Answer from the drawing. Dimensions are ordinates in mm from the lowest x, y and z of the part. A direction names the side the tool comes from. Coordinates: 2 decimals unless noted, no trailing zeros. Write each loop counter-clockwise with the first axis right and the second up, starting at its lowest first coordinate (ties: lowest second). Pieces come first, ordered by that corner, then holes. Notation, with made-up numbers: (26.25, 67.5) -> (40.25, 67.5) arc R18 ccw to (40.25, 78.5) -> close; hole circle Ø4 at (58, 36). An arc over 180 degrees is marked (long way). Return JSON: item names as keys, results as strings.
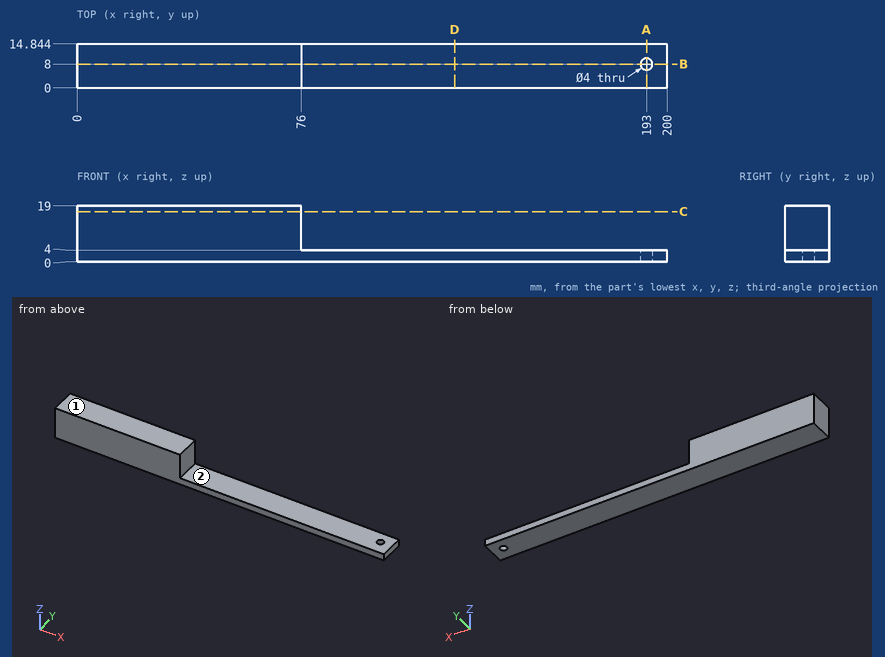
1. Consider L1, parallel to Y at x = 193, z = 1.6; L2, parallel to Z at x = 107, y = 10; L3, parallel to X at y = 1, z = 9. Determine where each line is inside the solid, lowest interval first.
Taken from the geometry:
{"L1": "y = 0 to 6, 10 to 14.84", "L2": "z = 0 to 4", "L3": "x = 0 to 76"}
2. The part is cut by section A-A (x = 193). Determine the outline of the cut face in (y, z).
Taken from the geometry:
{"outline": "(0, 0) -> (6, 0) -> (6, 4) -> (0, 4) -> close; (10, 0) -> (14.84, 0) -> (14.84, 4) -> (10, 4) -> close"}
3. A tool of negligible diameter and unlimited length cuts with its end or side. For the marked faces 1 and 2, from which of +Z, -Z, +X, -X, +Y, -Y can it reach the whole face along a straight path? Write none if from no direction.
Taken from the geometry:
{"face 1": "+Z, +X, -X, +Y, -Y", "face 2": "+Z, +X, +Y, -Y"}
4. The part is cut by section B-B (y = 8). Determine the outline of the cut face in (x, z), then the cut area to 3 significant figures.
Taken from the geometry:
{"outline": "(0, 0) -> (191, 0) -> (191, 4) -> (76, 4) -> (76, 19) -> (0, 19) -> close; (195, 0) -> (200, 0) -> (200, 4) -> (195, 4) -> close", "area": "1,920 mm2"}
5. The part is cut by section D-D (x = 128). Determine the outline of the cut face in (y, z).
Taken from the geometry:
{"outline": "(0, 0) -> (14.84, 0) -> (14.84, 4) -> (0, 4) -> close"}
6. Flat-ended cylindrical pins translate along their axes: pin 1 Ø1 at (y, z) = (7.5, 8) entering from +X; pin 2 Ø4.5 at (x, y) = (193, 8) entering from +Z; pin 3 Ø1.5 at (y, z) = (12, 3.5) entering from -X; pin 4 Ø1.5 at (x, z) = (141.5, 5) entering from +Y. Find the tip coordinate at first contact, or state that the pin passes through.
Taken from the geometry:
{"pin 1": "stops at x = 76", "pin 2": "stops at z = 4", "pin 3": "stops at x = 0", "pin 4": "passes through"}
7. The part is cut by section C-C (z = 17). Determine the outline of the cut face in (x, y).
Taken from the geometry:
{"outline": "(0, 0) -> (76, 0) -> (76, 14.84) -> (0, 14.84) -> close"}
